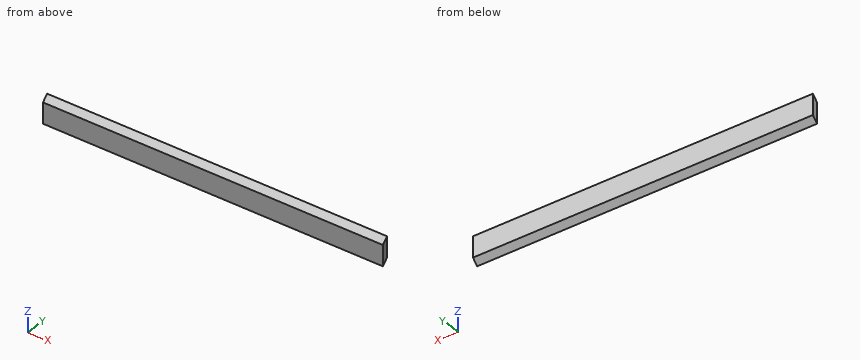
from build123d import *

# Parameters (mm, degrees)
F0_W     = 1181.1
F0_H     = 71.8312
F1_DEPTH = 19.05
F3_DEPTH = 1181.101
F5_DEPTH = 1181.1


with BuildPart() as f1:
    # F0 (on Front) → F1 (new body)
    with BuildSketch(Plane.XZ):
        Rectangle(F0_W, F0_H)
    extrude(amount=F1_DEPTH)

    # F2 (on face) → F3 (cut, through all)
    with BuildSketch(Plane.YZ.offset(590.55)):
        Polygon((0, -16.8656), (-19.05, -35.9156), (0, -35.9156), align=None)
    extrude(amount=-F3_DEPTH, mode=Mode.SUBTRACT)

    # F4 (on face) → F5 (join)
    with BuildSketch(Plane.YZ.offset(590.55)):
        Polygon((0, 54.9656), (-19.05, 35.9156), (0, 35.9156), align=None)
    extrude(amount=-F5_DEPTH)


solid = f1.part
Read the model definition and answer for the solid it produces. Units are mm, in the model's axes. Coordinates: 2 decimals unless noted, no trailing zeros. Order: outer loops, then holes, each group sorted by start corner. A loop starts at its lowest first (then second) coordinate and runs counter-clockwise, first axis right, second up. Notation, with made-up numbers: (-32.75, 61.25) - (5.25, 61.25) arc R14 ccw to (5.25, 69.25) - close; hole circle Ø5 at (71.25, -15.75). An arc over 180 degrees is marked (long way). Use one line per item in the form item = value.
(1) Given pin 1 Ø5 at (x, y) = (-218, -9.5) entering from -Z; pin 2 Ø1.5 at (x, y) = (-122, -12) entering from +Z, each flat-ended and moving along its own axis, determine where each tip first touches the part or whether it passes through.
Computed values:
pin_1 = -28.87
pin_2 = 43.72
(2) Section A-A, the plane x = 197 is taken. Give the vertices of the cut face in (y, z).
Computed values:
outline = (-19.05, -35.92) - (0, -16.87) - (0, 54.97) - (-19.05, 35.92) - close
(3) Section B-B, the plane y = -8 is taken. Give the vertices of the cut face in (x, z).
Computed values:
outline = (-590.55, -24.87) - (590.55, -24.87) - (590.55, 46.97) - (-590.55, 46.97) - close
(4) Straight lines are drawn through the part: L1, parallel to Y at x = 291.5, z = 36; L2, parallel to Y at x = -312, z = -20; L3, parallel to Z at x = -467, y = -7.5. For each, find the intervals that lie inside material, in ascending order.
Computed values:
L1 = -18.97 to 0
L2 = -19.05 to -3.13
L3 = -24.37 to 47.47
